Model file for the job. Use its own axes, mm. A direction names the side the tool comes from. Coordinates: 2 decimals unless noted, no trailing zeros. Loops run counter-clockwise (first coordinate to the right, second up) from the corner with the lowest first, then second, coordinate; pieces in that order, holes last.
Autodesk Inventor part; units mm, degrees
ref_plane "РабПлоскость1" through (10, 0, 150) normal (-1, 0, 0) x (0, 0, 1)
ref_plane "YZ Plane" through (0, 0, 0) normal (1, 0, 0) x (0, 1, 0)
ref_plane "XZ Plane" through (0, 0, 0) normal (0, 1, 0) x (-1, 0, 0)
sketch "Эскиз1" plane through (0, 0, 0) normal (0, 0, 1) x (1, 0, 0)
  line L0 (0, 0) -> (20, 0)
  line L1 (20, 0) -> (20, 20)
  line L2 (20, 20) -> (0, 20)
  line L3 (0, 20) -> (0, 0)
  line L4 (1.5, 1.5) -> (18.5, 1.5)
  line L5 (18.5, 1.5) -> (18.5, 18.5)
  line L6 (18.5, 18.5) -> (1.5, 18.5)
  line L7 (1.5, 18.5) -> (1.5, 1.5)
  point P0 (10, 18.5)
  point P1 (10, 20)
  point P2 (18.5, 10)
  point P3 (20, 10)
  dimension "d0" = 20
  dimension "d1" = 1.5
extrude "Выдавливание1" add sketch "Эскиз1" along normal blind 150
sketch "Эскиз3" plane through (0, 20, 0) normal (0, 1, 0) x (1, 0, 0)
  line L0 (0, 0) -> (0, -150)
  line L1 (0, -7) -> (-15, 0)
  line L2 (-15, 0) -> (0, 0)
  line L3 (0, 0) -> (0, -7)
  line L4 (0, -7) -> (0, 0)
  dimension "d4" = 15
  dimension "d5" = 7
extrude "Выдавливание2" add sketch "Эскиз3" against normal up to surface (20 mm away)
ref_plane "РабПлоскость1" through (10, 0, 150) normal (-1, 0, 0) x (0, 0, 1)
mirror "Зеркальное отражение1" about plane through (10, 0, 150) normal (-1, 0, 0) of "Выдавливание2"
properties part number "shock_absorber_holder"
Q1. Slice it at B-B (x = 14). List the corners of the cut face in (y, z), and give its area (3 significant figures).
Answers:
outline: (0, 0) - (1.5, 0) - (1.5, 150) - (0, 150) - close; (18.5, 0) - (20, 0) - (20, 150) - (18.5, 150) - close
area: 450 mm2
Q2. Slice it at D-D (x = 26). List the corners of the cut face in (y, z), and give its area (3 significant figures).
Answers:
outline: (0, 0) - (20, 0) - (20, 4.2) - (0, 4.2) - close
area: 84.0 mm2
Q3. Which spindle directions (+Z, -Z, +X, -X, +Y, -Y) get a long thin tool onto all of the face, cutting with end or side? Do faces 4 (the flat face through (20, 10, 77)), 5 (the flat face through (0, 10, 77)), 6 (the flat face through (1.5, 10, 74)). Say none if no direction does.
Answers:
face 4: +Z, +X, +Y, -Y
face 5: +Z, -X, +Y, -Y
face 6: +Z, -Z
Q4. Flat gauge pins, fed straight in: P1, Ø1, axis at y = 13.5, z = 26.5, coming from the +X side; P2, Ø12, axis at x = 28, y = 14.5, coming from the +Z side; P3, Ø2, axis at x = 27.5, y = 17.5, coming from the +Z side. Where does each tip first touch, or does it go through?
Answers:
P1: stops at x = 20
P2: stops at z = 6.07
P3: stops at z = 3.97
Q5. Mould opens along Y. For faces 1 (the flat face through (10, 1.5, 74)), 2 (the flat face through (10, 19, 0)), 3 (the flat face through (10, 0, 69)) say: +Y half, -Y half, draft (parallel to the pull), parting line (faces both ways), or undercut.
Answers:
face 1: undercut
face 2: draft
face 3: -Y half
Q6. Drill centre lines: line 1 (X direction, y = 10.75, z = 67.5); line 2 (Z direction, x = -2.5, y = 10.75). Where is each one in solid material? Low to high.
Answers:
line 1: x = 0 to 1.5, 18.5 to 20
line 2: z = 0 to 5.83
Q7. Slice it at C-C (z = 57). List the corners of the cut face in (x, y), and give its area (3 significant figures).
Answers:
outline: (0, 0) - (20, 0) - (20, 20) - (0, 20) - close; hole (1.5, 1.5) - (18.5, 1.5) - (18.5, 18.5) - (1.5, 18.5) - close
area: 111 mm2
Q8. Slice it at A-A (y = 4). List the corners of the cut face in (x, z), and give its area (3 significant figures).
Answers:
outline: (-15, 0) - (1.5, 0) - (1.5, 150) - (0, 150) - (0, 7) - close; (18.5, 0) - (35, 0) - (20, 7) - (20, 150) - (18.5, 150) - close
area: 555 mm2
